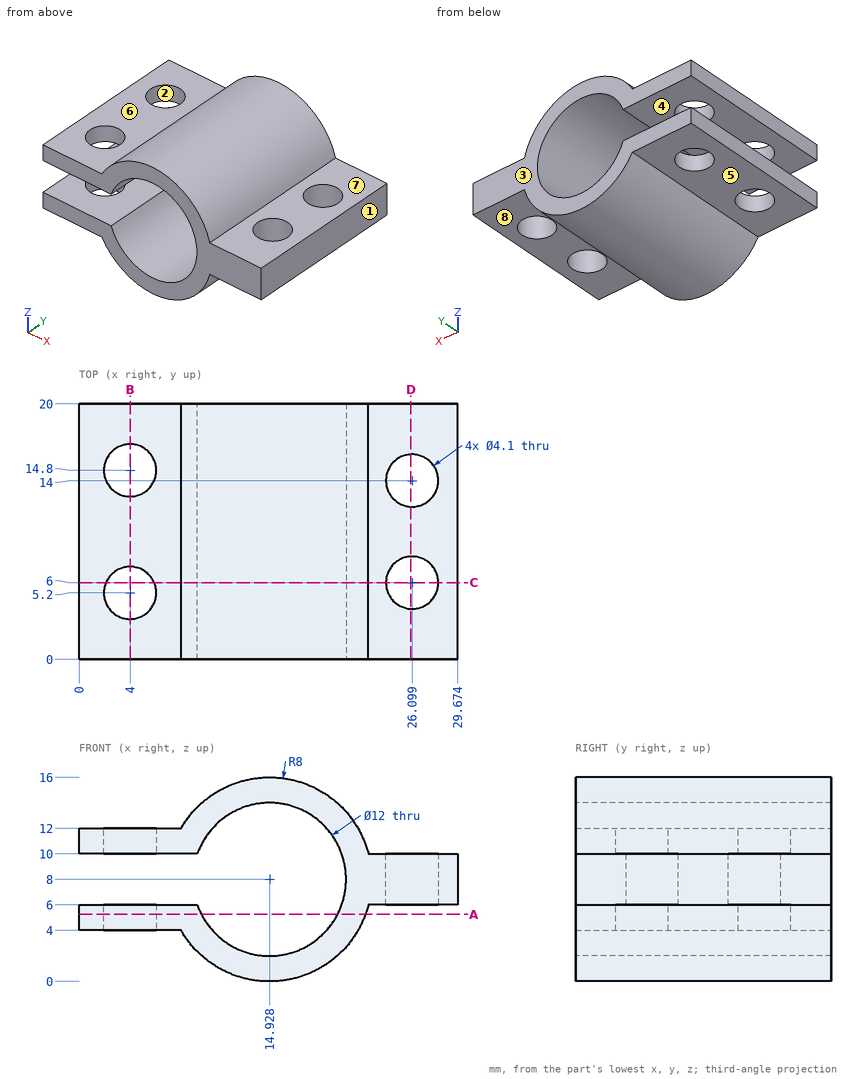
For this review, use the dimensioned drawing (mm, ordinates from the lowest corner) and the shaded views. A direction names the side the tool comes from. Give positions to 0.01 mm unless a question says otherwise; leave off trailing zeros. Loops run counter-clockwise (first coordinate to the right, second up) from the corner with the lowest first, then second, coordinate; pieces in that order, holes last. Notation, with made-up numbers: (-31, 55) - (10, 55) arc R23 ccw to (10, 84) - close; hole circle Ø4 at (6.5, -6). An arc over 180 degrees is marked (long way). Write each question's results on one line, items separated by ' | '.
(1) For line 1 along Y through (x, z) = (4, 10.55); line 2 along Z through (x, y) = (1.75, 13.5); line 3 along X through (y, z) = (4.25, 8.25) (1 decimal), list the stretches that pass through material, from the lowest coordinate up.
Conclusion:
line 1: 0 to 3.15, 7.25 to 12.75, 16.85 to 20 | line 2: 4 to 6, 10 to 12 | line 3: 20.9 to 25, 27.2 to 29.7
(2) Take a section at D-D (x = 26). Give the boundary of the cut face in (y, z).
Conclusion:
outline: (0, 6) - (3.95, 6) - (3.95, 10) - (0, 10) - close; (8.05, 6) - (11.95, 6) - (11.95, 10) - (8.05, 10) - close; (16.05, 6) - (20, 6) - (20, 10) - (16.05, 10) - close
(3) Take a section at C-C (y = 6). Give the boundary of the cut face in (x, z).
Conclusion:
outline: (0, 4) - (2.11, 4) - (2.11, 6) - (0, 6) - close; (0, 10) - (2.11, 10) - (2.11, 12) - (0, 12) - close; (5.89, 4) - (8, 4) arc R8 ccw to (22.67, 6) - (24.05, 6) - (24.05, 10) - (22.67, 10) arc R8 ccw to (8, 12) - (5.89, 12) - (5.89, 10) - (9.27, 10) arc R6 cw (long way) to (9.27, 6) - (5.89, 6) - close; (28.15, 6) - (29.67, 6) - (29.67, 10) - (28.15, 10) - close
(4) Take a section at A-A (z = 5.25). Give the boundary of the cut face in (x, y).
Conclusion:
outline: (0, 0) - (9.6, 0) - (9.6, 20) - (0, 20) - close; (20.26, 0) - (22.44, 0) - (22.44, 20) - (20.26, 20) - close; hole circle Ø4.1 at (4, 5.2); hole circle Ø4.1 at (4, 14.8)
(5) Take a section at B-B (x = 4). Give the boundary of the cut face in (y, z).
Conclusion:
outline: (0, 4) - (3.15, 4) - (3.15, 6) - (0, 6) - close; (0, 10) - (3.15, 10) - (3.15, 12) - (0, 12) - close; (7.25, 4) - (12.75, 4) - (12.75, 6) - (7.25, 6) - close; (7.25, 10) - (12.75, 10) - (12.75, 12) - (7.25, 12) - close; (16.85, 4) - (20, 4) - (20, 6) - (16.85, 6) - close; (16.85, 10) - (20, 10) - (20, 12) - (16.85, 12) - close
(6) Draft analysis for pull direction Y (two halves, no side actions). For the marked faces 1, 2 and 3, state which applies: +Y half, -Y half, draft (parallel to the pull), parting line (faces both ways), or undercut.
Conclusion:
face 1: draft | face 2: undercut | face 3: +Y half
(7) For the marked faces 4, 5, 6, 7 and 8, list the 3-axis set-ups (+Z, -Z, +X, -X, +Y, -Y) from which the entire face can be reached by the end or side of a thin tool; tool diameter is ignored.
Conclusion:
face 4: -X, +Y, -Y | face 5: -Z, -X, +Y, -Y | face 6: +Z, -X, +Y, -Y | face 7: +Z, +X, +Y, -Y | face 8: -Z, +X, +Y, -Y
(8) For pin 1 Ø6.5 at (x, y) = (4, 5.2) entering from +Z; pin 2 Ø10 at (x, y) = (5, 13.5) entering from +Z; pin 3 Ø5.5 at (x, y) = (25.5, 7.5) entering from -Z, all flat-tipped, find the tip position at first contact; note any pin that passes through.
Conclusion:
pin 1: z = 12 | pin 2: z = 14.3 | pin 3: z = 6
